```python
from build123d import *

# Parameters (mm, degrees)
SKETCH1_W               = 50.8
SKETCH1_H               = 50.8
BOSS_EXTRUDE1_DEPTH     = 69.85
SHELL1_T                = -3.175
SKETCH2_W               = 31.75
SKETCH2_H               = 26.9875
CUT_EXTRUDE1_DEPTH      = 79.545162168
FILLET1_R               = 3.175
CUT_EXTRUDE2_DEPTH      = 79.545162168
CUT_EXTRUDE2_DEPTH_BACK = 79.545162168
SKETCH3_R               = 3.175
CUT_EXTRUDE3_DEPTH      = 79.545162168
CUT_EXTRUDE3_DEPTH_BACK = 79.545162168
SKETCH4_R               = 2.4892
CUT_EXTRUDE4_DEPTH      = 79.545162168
CUT_EXTRUDE4_DEPTH_BACK = 79.545162168
SKETCH5_R               = 2.4892
FILLET2_R               = 3.175
SKETCH6_W               = 139.7
SKETCH6_H               = 47.625
CUT_EXTRUDE5_DEPTH      = 91.02678768


with BuildPart() as part:
    # Sketch1 → Boss-Extrude1 (new, symmetric)
    with BuildSketch(Plane.XY):
        Rectangle(SKETCH1_W, SKETCH1_H)
    extrude(amount=BOSS_EXTRUDE1_DEPTH, both=True)

    # Shell1
    shell1_openings = [part.faces().sort_by_distance(p)[0] for p in [
        (0, 0, 69.85),
        (0, 0, -69.85),
    ]]
    offset(amount=SHELL1_T, openings=shell1_openings, kind=Kind.INTERSECTION)

    # Sketch2 → Cut-Extrude1 (cut, through all)
    with BuildSketch(Plane(origin=(0, 0, 0), x_dir=(1, 0, 0), z_dir=(0, 1, 0))):
        with Locations((0, 31.75)):
            Rectangle(SKETCH2_W, SKETCH2_H)
        with Locations((0, -47.625)):
            Rectangle(SKETCH2_W, SKETCH2_H)
    extrude(amount=CUT_EXTRUDE1_DEPTH, mode=Mode.SUBTRACT)

    # Fillet1
    fillet1_edges = [part.edges().sort_by_distance(p)[0] for p in [
        (15.875, 23.8125, -18.25625),
        (15.875, 23.8125, -45.24375),
        (-15.875, 23.8125, -45.24375),
        (-15.875, 23.8125, -18.25625),
    ]]
    fillet(fillet1_edges, radius=FILLET1_R)

    # Sketch3 → Cut-Extrude2 (cut, two sides: drawn at the far end of the back side and taken through both)
    with BuildSketch(Plane(origin=(0, 0, 0), x_dir=(0, 0, -1), z_dir=(1, 0, 0)).offset(-CUT_EXTRUDE2_DEPTH_BACK)):
        with Locations((31.75, 9.525)):
            Circle(SKETCH3_R)
        with Locations((-44.45, 9.525)):
            Circle(SKETCH3_R)
    extrude(amount=CUT_EXTRUDE2_DEPTH + CUT_EXTRUDE2_DEPTH_BACK, mode=Mode.SUBTRACT)

    # Sketch4 → Cut-Extrude3 (cut, two sides: drawn at the far end of the back side and taken through both)
    with BuildSketch(Plane(origin=(0, 0, 0), x_dir=(0, 0, -1), z_dir=(1, 0, 0)).offset(-CUT_EXTRUDE3_DEPTH_BACK)):
        with Locations((57.15, 12.7)):
            Circle(SKETCH4_R)
        with Locations((44.45, -12.7)):
            Circle(SKETCH4_R)
        with Locations((31.75, -12.7)):
            Circle(SKETCH4_R)
        with Locations((19.05, -12.7)):
            Circle(SKETCH4_R)
        with Locations((57.15, 0)):
            Circle(SKETCH4_R)
        with Locations((57.15, -12.7)):
            Circle(SKETCH4_R)
        with Locations((-61.9125, 12.7)):
            Circle(SKETCH4_R)
        with Locations((-11.1125, 12.7)):
            Circle(SKETCH4_R)
        with Locations((-36.5125, -12.7)):
            Circle(SKETCH4_R)
        with Locations((-11.1125, -12.7)):
            Circle(SKETCH4_R)
        with Locations((-61.9125, -12.7)):
            Circle(SKETCH4_R)
    extrude(amount=CUT_EXTRUDE3_DEPTH + CUT_EXTRUDE3_DEPTH_BACK, mode=Mode.SUBTRACT)

    # Sketch5 → Cut-Extrude4 (cut, two sides: drawn at the far end of the back side and taken through both)
    with BuildSketch(Plane(origin=(0, 0, 0), x_dir=(1, 0, 0), z_dir=(0, 1, 0)).offset(-CUT_EXTRUDE4_DEPTH_BACK)):
        with Locations(Location((-12.7, -57.15, 0), (0, 0, 270))):
            Circle(SKETCH5_R)
        with Locations(Location((0, -57.15, 0), (0, 0, 270))):
            Circle(SKETCH5_R)
        with Locations(Location((12.7, -57.15, 0), (0, 0, 270))):
            Circle(SKETCH5_R)
    extrude(amount=CUT_EXTRUDE4_DEPTH + CUT_EXTRUDE4_DEPTH_BACK, mode=Mode.SUBTRACT)

    # Fillet2
    fillet2_edges = [part.edges().sort_by_distance(p)[0] for p in [
        (15.875, 23.8125, 61.11875),
        (15.875, 23.8125, 34.13125),
        (-15.875, 23.8125, 34.13125),
        (-15.875, 23.8125, 61.11875),
    ]]
    fillet(fillet2_edges, radius=FILLET2_R)

    # Sketch6 → Cut-Extrude5 (cut, through all)
    with BuildSketch(Plane(origin=(25.4, 0, 0), x_dir=(0, 0, -1), z_dir=(1, 0, 0))):
        with Locations((0, -1.5875)):
            Rectangle(SKETCH6_W, SKETCH6_H)
    extrude(amount=-CUT_EXTRUDE5_DEPTH, mode=Mode.SUBTRACT)


solid = part.part
```
Part model, mm, in its own coordinate system. A direction names the side the tool comes from. Coordinates: 2 decimals unless noted, no trailing zeros. Order: outer loops, then holes, each group sorted by start corner. A loop starts at its lowest first (then second) coordinate and runs counter-clockwise, first axis right, second up. Notation, with made-up numbers: (45.25, -1) - (57.25, -1) arc R27 ccw to (57.25, 37) - close; hole circle Ø7 at (-32, 21). An arc over 180 degrees is marked (long way). Return JSON: item names as keys, results as strings. Group by question number.
Item 1: Drill centre lines: probe 1 along Z at (x, y) = (0, 24.35); probe 2 along X at (y, z) = (22.9, -24) (3 decimals); probe 3 along Z at (x, y) = (15.5, 23). Where is each one in solid material? Low to high. Write a range as from..to.
Item 2: Pull direction Z, two halves, no side cores. Call faces 1 (the face through (25.4, 24, 1)), 2 (the face through (14.92, 23.83, -44.34)), 3 (the face through (-14.97, 23.83, -19.21)), 4 (the face through (0, 24, 69.85)): pulls with the +Z half, pulls with the -Z half, needs draft (parallel to the pull), parting line crosses it, or undercut.
Item 3: Which spindle directions (+Z, -Z, +X, -X, +Y, -Y) get a long thin tool onto all of the face, cutting with end or side? Do faces 5 (the face through (0, 24, 34.131)), 6 (the face through (0, 22.225, 1)). Say none if no direction does.
Item 4: Cut at B-B (y = 23.4). List the corners of the cut face in (x, z) (3 decimals).
Item 5: Cut at D-D (x = -14.5). List the corners of the cut face in (y, z) (3 decimals).
Item 6: Cut at C-C (z = -33). List the corners of the cut face in (x, y) (3 decimals).
Item 7: Cut at A-A (x = 7.5). List the corners of the cut face in (y, z) (3 decimals), plus the area to 3 significant figures.
Check values:
{
 "1": {"probe 1": "z = -69.85..-45.24, -18.26..34.13, 61.12..69.85", "probe 2": "x = -25.4..-15.875, 15.875..25.4", "probe 3": "z = -69.85..-43.57, -19.93..35.81, 59.44..69.85"},
 "2": {"face 1": "needs draft", "face 2": "undercut", "face 3": "undercut", "face 4": "pulls with the +Z half"},
 "3": {"face 5": "+Y, -Y", "face 6": "+Z, -Z, +X, -X, -Y"},
 "4": {"outline": "(-25.4, -69.85) - (25.4, -69.85) - (25.4, 69.85) - (-25.4, 69.85) - close; hole (-15.875, -42.069) arc R3.175 ccw to (-12.7, -45.244) - (12.7, -45.244) arc R3.175 ccw to (15.875, -42.069) - (15.875, -21.431) arc R3.175 ccw to (12.7, -18.256) - (-12.7, -18.256) arc R3.175 ccw to (-15.875, -21.431) - close; hole (-15.875, 37.306) arc R3.175 ccw to (-12.7, 34.131) - (12.7, 34.131) arc R3.175 ccw to (15.875, 37.306) - (15.875, 57.944) arc R3.175 ccw to (12.7, 61.119) - (-12.7, 61.119) arc R3.175 ccw to (-15.875, 57.944) - close"},
 "5": {"outline": "(22.225, -69.85) - (25.4, -69.85) - (25.4, -44.684) - (22.225, -44.684) - close; (22.225, -18.816) - (25.4, -18.816) - (25.4, 34.691) - (22.225, 34.691) - close; (22.225, 60.559) - (25.4, 60.559) - (25.4, 69.85) - (22.225, 69.85) - close"},
 "6": {"outline": "(-25.4, 22.225) - (-15.875, 22.225) - (-15.875, 25.4) - (-25.4, 25.4) - close; (15.875, 22.225) - (25.4, 22.225) - (25.4, 25.4) - (15.875, 25.4) - close"},
 "7": {"outline": "(22.225, -69.85) - (25.4, -69.85) - (25.4, -45.244) - (22.225, -45.244) - close; (22.225, -18.256) - (25.4, -18.256) - (25.4, 34.131) - (22.225, 34.131) - close; (22.225, 61.119) - (25.4, 61.119) - (25.4, 69.85) - (22.225, 69.85) - close", "area": "272 mm2"}
}
